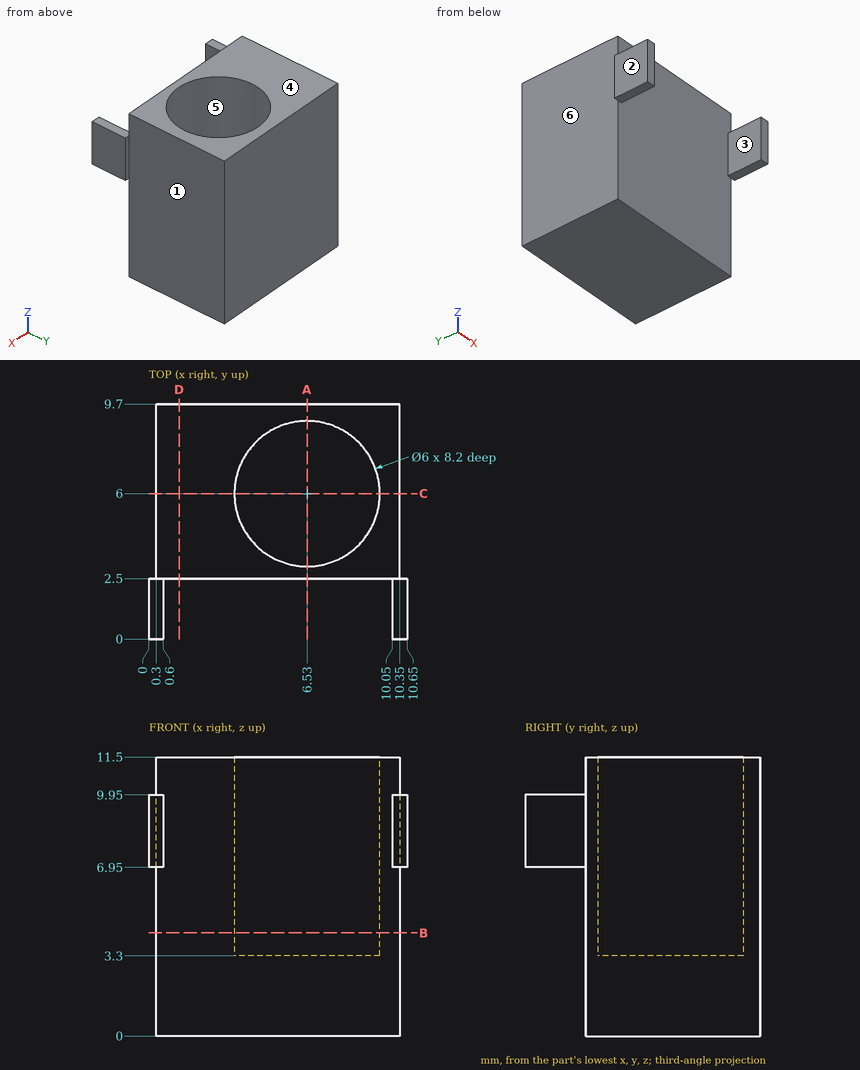
Design review of the part shown in the three views and the two pictorial views. Dimensions are in mm from the part's minimum x, y and z. A direction names the side the tool comes from. Coordinates: 2 decimals unless noted, no trailing zeros. Loops run counter-clockwise (first coordinate to the right, second up) from the corner with the lowest first, then second, coordinate; pieces in that order, holes last. Notation, with made-up numbers: (82.25, -24) - (117.25, -24) arc R23 cw to (117.25, 3) - close; hole circle Ø5 at (-5, 53). An arc over 180 degrees is marked (long way). Use a Markdown table: item, result. Add a question column.
Item 1: We need section D-D (x = 1.25). Give the boundary of the cut face in (y, z).
Item 2: We need section B-B (z = 4.25). Give the boundary of the cut face in (x, y), and give its area (3 significant figures).
Item 3: We need section A-A (x = 6.53). Give the boundary of the cut face in (y, z), and give its area (3 significant figures).
Item 4: We need section C-C (y = 6). Give the boundary of the cut face in (x, z).
Item 5: Tool access review of the marked faces 1, 2 and 3: name each direction out of +Z, -Z, +X, -X, +Y, -Y from which nothing blocks a thin tool from reaching the whole face with its end or side.
Item 6: Mouldability with a two-part tool opening along X and no side actions: class the marked faces 4, 5 and 6 as pulls with the +X half, pulls with the -X half, needs draft (parallel to the pull), parting line crosses it, or undercut.
Item 7: Insertion check: pin 1 Ø2 at (y, z) = (8.5, 9) entering from -X; pin 2 Ø5 at (x, y) = (7, 4.5) entering from -Z; pin 3 Ø1.5 at (y, z) = (7, 8) entering from +X; pin 4 Ø5 at (x, z) = (5, 5.5) entering from -Y. Each pin has a flat end and moves straight along its axis. Give the tip position at first contact, or say it passes through.
Item 8: For line 1 (Y direction, x = 6.53, z = 7.75); line 2 (Z direction, x = 6.5, y = 5.25); line 3 (X direction, y = 4.75, z = 6.25), list the stretches that pass through material, from the lowest coordinate up.
Results list:
| question | item | result |
|---|---|---|
| 1 | outline | (2.5, 0) - (9.7, 0) - (9.7, 11.5) - (2.5, 11.5) - close |
| 2 | outline | (0.3, 2.5) - (10.35, 2.5) - (10.35, 9.7) - (0.3, 9.7) - close; hole circle Ø6 at (6.53, 6) |
| 2 | area | 44.1 mm^2 |
| 3 | outline | (2.5, 0) - (9.7, 0) - (9.7, 11.5) - (9, 11.5) - (9, 3.3) - (3, 3.3) - (3, 11.5) - (2.5, 11.5) - close |
| 3 | area | 33.6 mm^2 |
| 4 | outline | (0.3, 0) - (10.35, 0) - (10.35, 11.5) - (9.53, 11.5) - (9.53, 3.3) - (3.53, 3.3) - (3.53, 11.5) - (0.3, 11.5) - close |
| 5 | face 1 | +Z, -Z, +X, +Y |
| 5 | face 2 | +Z, -Z, -X, +Y, -Y |
| 5 | face 3 | +Z, -Z, -Y |
| 6 | face 4 | needs draft |
| 6 | face 5 | undercut |
| 6 | face 6 | pulls with the -X half |
| 7 | pin 1 | stops at x = 0.3 |
| 7 | pin 2 | stops at z = 0 |
| 7 | pin 3 | stops at x = 10.35 |
| 7 | pin 4 | stops at y = 2.5 |
| 8 | line 1 | y = 2.5 to 3, 9 to 9.7 |
| 8 | line 2 | z = 0 to 3.3 |
| 8 | line 3 | x = 0.3 to 3.8, 9.26 to 10.35 |
